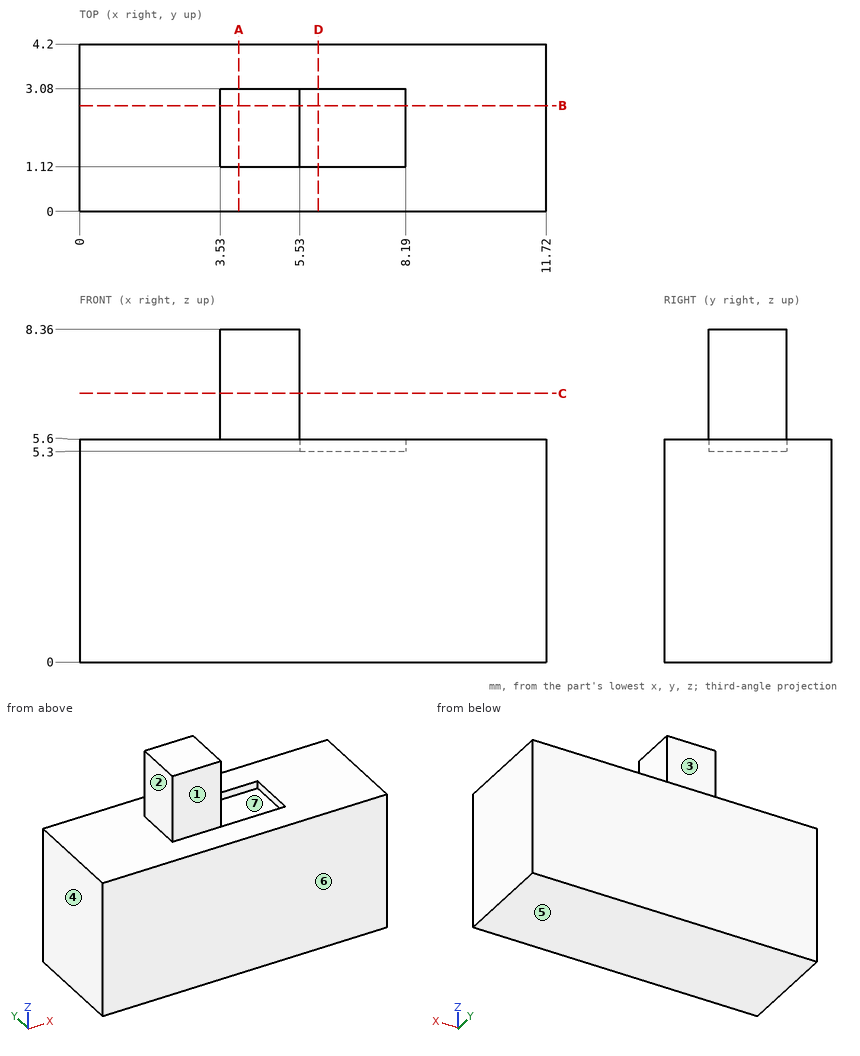
Here's the drawing with two shaded views (mm, measured from the low corner). I have some questions. A direction names the side the tool comes from. Coordinates: 2 decimals unless noted, no trailing zeros. Order: outer loops, then holes, each group sorted by start corner. A loop starts at its lowest first (then second) coordinate and runs counter-clockwise, first axis right, second up.
Item 1: Which directions (+Z, -Z, +X, -X, +Y, -Y) give clear straight access to the entire face, cutting with the end or side of a thin tool? Please do the marked faces 1, 2, 3 and 4.
Response values:
face 1: +Z, +X, -X, -Y
face 2: +Z, -X, +Y, -Y
face 3: +Z, +X, -X, +Y
face 4: +Z, -Z, -X, +Y, -Y
Item 2: If we section it at B-B, the plane y = 2.65: List the corners of the cut face in (x, z) for me, then the cut area to 3 significant figures.
Response values:
outline: (0, 0) - (11.72, 0) - (11.72, 5.6) - (8.19, 5.6) - (8.19, 5.3) - (5.53, 5.3) - (5.53, 8.36) - (3.53, 8.36) - (3.53, 5.6) - (0, 5.6) - close
area: 70.4 mm2
Item 3: Thinking about a two-plate mould opening in Y: for the marked faces 5, 6 and 7, which applies, pulls with the +Y half, pulls with the -Y half, needs draft (parallel to the pull), parting line crosses it, or undercut?
Response values:
face 5: needs draft
face 6: pulls with the -Y half
face 7: undercut
Item 4: If we section it at C-C, the plane z = 6.75: List the corners of the cut face in (x, y) for me, then the cut area to 3 significant figures.
Response values:
outline: (3.53, 1.12) - (5.53, 1.12) - (5.53, 3.08) - (3.53, 3.08) - close
area: 3.92 mm2
Item 5: If we section it at D-D, the plane x = 6: List the corners of the cut face in (y, z) for me, then the cut area to 3 significant figures.
Response values:
outline: (0, 0) - (4.2, 0) - (4.2, 5.6) - (3.08, 5.6) - (3.08, 5.3) - (1.12, 5.3) - (1.12, 5.6) - (0, 5.6) - close
area: 22.9 mm2
Item 6: If we section it at A-A, the plane x = 4: List the corners of the cut face in (y, z) for me, then the cut area to 3 significant figures.
Response values:
outline: (0, 0) - (4.2, 0) - (4.2, 5.6) - (3.08, 5.6) - (3.08, 8.36) - (1.12, 8.36) - (1.12, 5.6) - (0, 5.6) - close
area: 28.9 mm2
Item 7: I need wall thicknesses on probe 1 along Z at (x, y) = (11, 3.25); probe 2 along Z at (x, y) = (7.75, 1.4); probe 3 along X at (y, z) = (1.5, 6.25). Which ranges of each line are inside material? Lowest first, please.
Response values:
probe 1: z = 0 to 5.6
probe 2: z = 0 to 5.3
probe 3: x = 3.53 to 5.53
Item 8: I'm going to push flat-ended pins straight in: pin 1 Ø2 at (x, z) = (4, 7.5) entering from +Y; pin 2 Ø0.6 at (x, z) = (4.5, 7) entering from -Y; pin 3 Ø1.6 at (y, z) = (2.5, 6.5) entering from +X. Where does each tip first touch, or does it pass through?
Response values:
pin 1: stops at y = 3.08
pin 2: stops at y = 1.12
pin 3: stops at x = 5.53
